```python
from build123d import *

# Parameters (mm, degrees)
SKETCH_1_R          = 49.855
EXTRUDE_1_DEPTH     = 95.18
SKETCH_3_R          = 15
SKETCH_4_R          = 15
CUT_EXTRUDE_1_DEPTH = 250
CHAMFER_1_SIZE      = 3
FILLET_1_R          = 5


with BuildPart() as part:
    # 草图1 → 凸台-拉伸1 (new body)
    with BuildSketch(Plane(origin=(0, 513.97, 0), x_dir=(1, 0, 0), z_dir=(0, 1, 0))):
        with Locations(Location((-989.291415846, 54.73, 0), (0, 0, 90))):
            Circle(SKETCH_1_R)
    extrude(amount=EXTRUDE_1_DEPTH)

    # 草图3 → 切除-旋转1 (revolve, cut)
    with BuildSketch(Plane.XY.offset(-54.73), mode=Mode.PRIVATE) as cut_revolve_1_sk:
        with Locations((-1049.146415846, 561.56)):
            Circle(SKETCH_3_R)
    revolve(cut_revolve_1_sk.sketch.rotate(Axis((-989.291415846, 609.15, -54.73), (0, -1, 0)), 90), axis=Axis((-989.291415846, 609.15, -54.73), (0, -1, 0)), mode=Mode.SUBTRACT)

    # 草图4 → 切除-拉伸1 (cut, symmetric)
    with BuildSketch(Plane(origin=(0, 609.15, 0), x_dir=(1, 0, 0), z_dir=(0, 1, 0))):
        with Locations(Location((-989.291415846, 54.73, 0), (0, 0, 270))):
            Circle(SKETCH_4_R)
    extrude(amount=CUT_EXTRUDE_1_DEPTH, both=True, mode=Mode.SUBTRACT)

    # 倒角1
    chamfer_1_edges = [part.edges().sort_by_distance(p)[0] for p in [
        (-989.291415846, 609.15, -69.73),
        (-989.291415846, 513.97, -69.73),
    ]]
    chamfer(chamfer_1_edges, length=CHAMFER_1_SIZE)

    # 圆角1
    fillet_1_edges = [part.edges().sort_by_distance(p)[0] for p in [
        (-989.291415846, 513.97, -4.875),
        (-989.291415846, 609.15, -4.875),
    ]]
    fillet(fillet_1_edges, radius=FILLET_1_R)


solid = part.part
```
The listing builds one solid part. Answer for the finished solid, in the listing's coordinates (mm). Coordinates: 2 decimals unless noted, no trailing zeros. Loops run counter-clockwise (first coordinate to the right, second up) from the corner with the lowest first, then second, coordinate; pieces in that order, holes last. Notation, with made-up numbers: M 17.5,-19.5 L 56.5,-19.5 A22 cw 56.5,-2.5 Z; hole C 88,-35.5 d3. An arc over 180 degrees is marked long. Answer as a JSON object with one key per item and string values. Group by question number.
Item 1: Determine the mould class of faces 1 (the face through (-1031.33, 534.45, -81.53)), 2 (the face through (-970, 609.15, -54)), 3 (the face through (-974.23, 606.34, -56.71)) for opening direction Z: +Z half, -Z half, draft (parallel to the pull), parting line (faces both ways), or undercut.
Item 2: Section A-A (z = -54.73) is taken. Write down the section's boundary in (x, y), and give its area (3 significant figures).
Item 3: Each of these flat-tipped pins is pushed along its axis until it touches: P1, Ø8, axis at x = -980, y = 547, coming from the +Z side; P2, Ø10, axis at y = 574.5, z = -20.5, coming from the +X side; P3, Ø24, axis at x = -989.29, z = -54.73, coming from the +Y side; P4, Ø6, axis at x = -978, y = 571.5, coming from the -Z side. Where does it stop, or does it pass through?
Item 4: Section B-B (y = 559) is taken. Write down the section's boundary in (x, z), and give its area (3 significant figures).
Item 5: Consider L1, parallel to X at y = 562, z = -54.73; L2, parallel to X at y = 585, z = -54.73; L3, parallel to Y at x = -1013.5, z = -15.5. Determine where each line is inside the solid, lowest interval first.
Solved:
{
 "1": {"face 1": "parting line", "face 2": "draft", "face 3": "undercut"},
 "2": {"outline": "M -1039.15,518.97 A5 ccw -1034.15,513.97 L -1007.29,513.97 L -1004.29,516.97 L -1004.29,606.15 L -1007.29,609.15 L -1034.15,609.15 A5 ccw -1039.15,604.15 L -1039.15,572.74 A15 cw -1039.15,550.38 Z; M -974.29,516.97 L -971.29,513.97 L -944.44,513.97 A5 ccw -939.44,518.97 L -939.44,550.38 A15 cw -939.44,572.74 L -939.44,604.15 A5 ccw -944.44,609.15 L -971.29,609.15 L -974.29,606.15 Z", "area": "6,440 mm2"},
 "3": {"P1": "stops at z = -5.16", "P2": "stops at x = -948.9", "P3": "passes through", "P4": "stops at z = -103.84"},
 "4": {"outline": "C -989.29,-54.73 d90.15; hole C -989.29,-54.73 d30", "area": "5,680 mm2"},
 "5": {"L1": "x = -1034.15 to -1004.29, -974.29 to -944.43", "L2": "x = -1039.15 to -1004.29, -974.29 to -939.44", "L3": "y = 514.13 to 555.58, 567.54 to 608.99"}
}
